The figure shows three views and two pictorial views of one solid part (mm, origin at its lowest corner). Answer the questions. Give positions to 0.01 mm unless a question says otherwise; leave off trailing zeros. Write each loop counter-clockwise with the first axis right and the second up, starting at its lowest first coordinate (ties: lowest second). Pieces come first, ordered by that corner, then holes. Notation, with made-up numbers: M 54,61.25 L 113,61.25 A17 cw 113,76.25 Z; hole C 12.25,75 d10. An arc over 180 degrees is marked long. Answer as CSV lines item,"result". Start each with the question number.
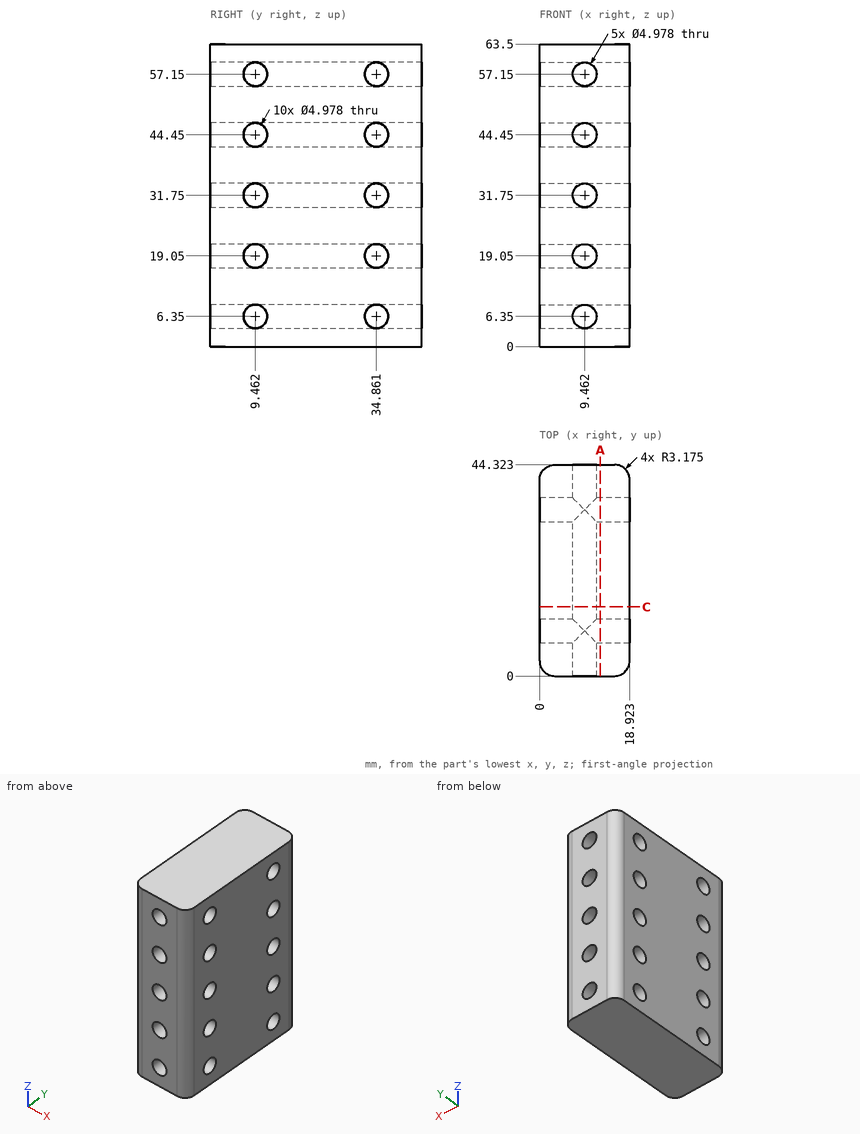
1. Find the intervals of material crossed by line 1 (Y direction, x = 3.5, z = 31.75); line 2 (Z direction, x = 9.5, y = 30); line 3 (Y direction, x = 16.5, z = 19.05), in increasing order. Write a range as [from, to].
2. Find section C-C on y = 14.5. Determine the outline of the cut face in (x, z), then the cut area to 3 significant figures.
3. Given pin 1 (3 mm diameter, centred on x = 9.46, z = 6.35, fed in from -Y), flat-ended and moving along its own axis, determine where the tip first touches the part or whether it passes through.
4. Find section A-A on x = 12.75. State how many separate pieces and enclosed holes the cut face has, then the cut area to 3 significant figures.
Computed:
1,line 1,"y = [0, 6.97], [11.95, 32.37], [37.35, 44.32]"
1,line 2,"z = [0, 3.86], [8.84, 16.56], [21.54, 29.26], [34.24, 41.96], [46.94, 54.66], [59.64, 63.5]"
1,line 3,"y = [0.09, 6.97], [11.95, 32.37], [37.35, 44.23]"
2,outline,"M 0,0 L 18.92,0 L 18.92,63.5 L 0,63.5 Z; hole C 9.46,6.35 d4.98; hole C 9.46,19.05 d4.98; hole C 9.46,31.75 d4.98; hole C 9.46,44.45 d4.98; hole C 9.46,57.15 d4.98"
2,area,"1,100 mm^2"
3,pin 1,"passes through"
4,separate pieces,"1"
4,enclosed holes,"10"
4,area,"2,620 mm^2"
